Study the drawing (mm; zero at the part's minimum x, y, z) and answer. A direction names the side the tool comes from. Coordinates: 2 decimals unless noted, no trailing zeros. Loops run counter-clockwise (first coordinate to the right, second up) from the corner with the lowest first, then second, coordinate; pieces in that order, holes last. Notation, with made-up numbers: (51, 17.5) -> (80, 17.5) arc R21 ccw to (80, 48.5) -> close; hole circle Ø6 at (7.25, -9.75). An arc over 180 degrees is marked (long way). Answer in a Markdown table with one row per item.
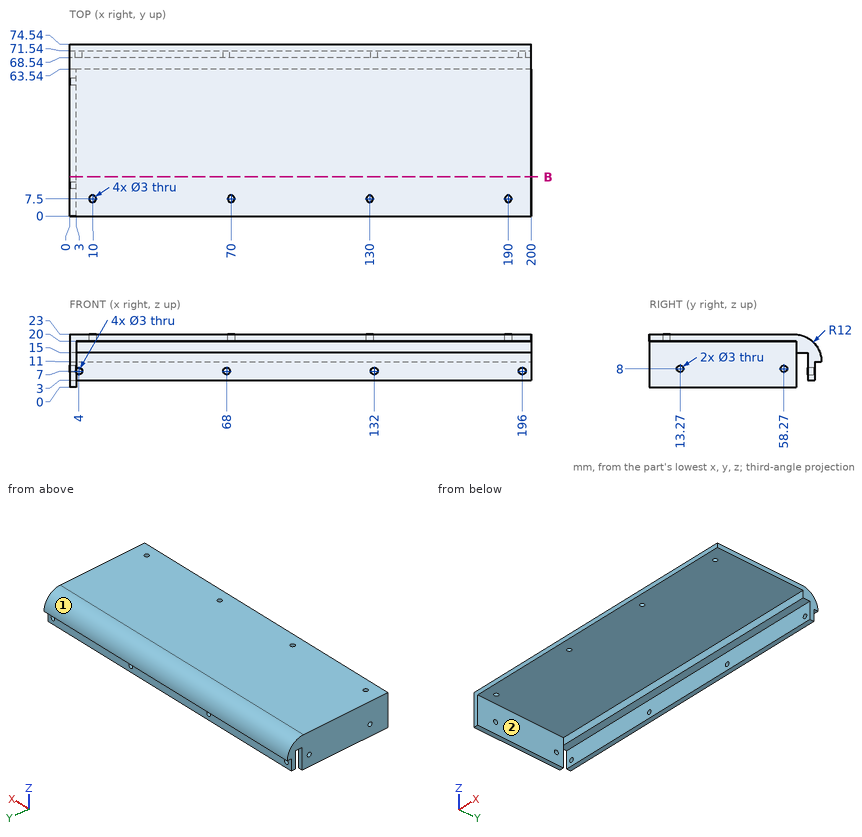
1. A cutting plane is placed at B-B on y = 17. Give the vertices of the cut face in (x, z), and give its area (3 significant figures).
A:
| item | result |
|---|---|
| outline | (0, 0) -> (3, 0) -> (3, 20) -> (200, 20) -> (200, 23) -> (0, 23) -> close |
| area | 660 mm2 |
2. A tool of negligible diameter and unlimited length cuts with its end or side. For the marked faces 1 and 2, from which of +Z, -Z, +X, -X, +Y, -Y can it reach the whole face along a straight path? Write none if from no direction.
A:
| item | result |
|---|---|
| face 1 | +Z, +X, -X, +Y |
| face 2 | -Z, +X, -Y |
3. Find the intervals of material crossed by probe 1 along X at (y, z) = (70.2, 7); probe 2 along Y at (x, z) = (1.3, 8); probe 3 along X at (y, z) = (36.5, 6.5), in increasing order.
A:
| item | result |
|---|---|
| probe 1 | x = 0 to 2.5, 5.5 to 66.5, 69.5 to 130.5, 133.5 to 194.5, 197.5 to 200 |
| probe 2 | y = 0 to 11.77, 14.77 to 56.77, 59.77 to 63.54, 68.54 to 71.54 |
| probe 3 | x = 0 to 3 |
4. Given pin 1 Ø1.5 at (x, z) = (64, 19.5) entering from +Y; pin 2 Ø3.5 at (y, z) = (13.27, 8) entering from +X; pin 3 Ø9.5 at (x, z) = (97, 8.5) entering from -Y; pin 4 Ø2.5 at (x, y) = (10, 7.5) entering from +Z (1 decimal), each flat-ended and moving along its own axis, determine where each tip first touches the part or whether it passes through.
A:
| item | result |
|---|---|
| pin 1 | stops at y = 71.7 |
| pin 2 | stops at x = 3 |
| pin 3 | stops at y = 68.54 |
| pin 4 | passes through |
